from build123d import *

# Parameters (mm, degrees)
BOSS_EXTRUDE2_DEPTH = 15
SKETCH4_R           = 5
BOSS_EXTRUDE3_DEPTH = 55
SKETCH5_R           = 2.5
BOSS_EXTRUDE5_DEPTH = 30
BOSS_EXTRUDE6_START = 20
SKETCH6_R           = 5
BOSS_EXTRUDE6_DEPTH = 20
SKETCH9_R           = 5
BOSS_EXTRUDE7_DEPTH = 20
SKETCH10_R          = 5
SKETCH10_R_2        = 3.5
CUT_EXTRUDE1_DEPTH  = 7


# Read off the part's stored shape, not the designer's step: Boss-Extrude2
with BuildPart() as part:
    # Boss-Extrude2 outline → Boss-Extrude2 (new body)
    with BuildSketch(Plane(origin=(0, 0, 0), x_dir=(1, 0, 0), z_dir=(0, 1, 0))):
        with BuildLine():
            ThreePointArc((-79.301270189, 80.000000278), (-85.640172505, 84.817399775), (-88.584206568, 77.419989152))
            add(Edge.make_bspline(
                [(-88.584206568, 77.419989152), (-86.367928891, 69.782262616), (-83.408582461, 63.514951385)],
                knots=[0.02157692, 0.02157692, 0.02157692, 0.151234515, 0.151234515, 0.151234515], degree=2))
            Line((-83.408582461, 63.514951385), (-110.262794416, 79.019237886))
            Line((-110.262794416, 79.019237886), (-115.262794416, 70.358983849))
            Line((-115.262794416, 70.358983849), (-63.301270189, 40.358983849))
            add(Edge.make_bspline(
                [(-63.301270189, 40.358983849), (-45.646570728, 30.396854404), (-18.218994006, 38.458495307)],
                knots=[0.484299762, 0.484299762, 0.484299762, 0.954512817, 0.954512817, 0.954512817], degree=2))
            ThreePointArc((-18.218994006, 38.458495307), (-3.922368216, 28.792616834), (12.885706155, 32.705589052))
            add(Edge.make_bspline(
                [(29.05383915, 7.474920109), (25.9728438, 20.230319759), (12.885706155, 32.705589052)],
                knots=[0.594463111, 0.594463111, 0.594463111, 0.969398026, 0.969398026, 0.969398026], degree=2))
            ThreePointArc((29.05383915, 7.474920109), (29.76251984, 3.767281878), (30, 0))
            add(Edge.make_bspline(
                [(13.669872981, -33.676914536), (30.204968933, -16.604131181), (30, 0)],
                knots=[0, 0, 0, 0.484954637, 0.484954637, 0.484954637], degree=2))
            ThreePointArc((13.669872981, -33.676914536), (12.667333455, -41.575264764), (20.545696107, -40.426167838))
            add(Edge.make_bspline(
                [(20.545696107, -40.426167838), (26.052022476, -34.6879518), (30, -28.991426998)],
                knots=[0.02157692, 0.02157692, 0.02157692, 0.151234515, 0.151234515, 0.151234515], degree=2))
            Line((30, -28.991426998), (30, -60))
            Line((30, -60), (40, -60))
            Line((40, -60), (40, 0))
            add(Edge.make_bspline(
                [(40, 0), (39.800107444, 20.270482952), (19.104733265, 39.992640706)],
                knots=[0.484299762, 0.484299762, 0.484299762, 0.954512817, 0.954512817, 0.954512817], degree=2))
            ThreePointArc((19.104733265, 39.992640706), (20.327316677, 57.206821065), (8.534546147, 69.80655435))
            add(Edge.make_bspline(
                [(65.631397208, 103.676914536), (19.549675952, 115.237660492), (8.534546147, 69.80655435)],
                knots=[0, 0, 0, 0.969398026, 0.969398026, 0.969398026], degree=2))
            ThreePointArc((65.631397208, 103.676914536), (72.972838916, 106.757864952), (68.038510461, 113.006178686))
            add(Edge.make_bspline(
                [(68.038510461, 113.006178686), (60.315906416, 114.905689184), (53.408582461, 115.476475612)],
                knots=[0.02157692, 0.02157692, 0.02157692, 0.151234515, 0.151234515, 0.151234515], degree=2))
            Line((53.408582461, 115.476475612), (80.262794416, 130.980762114))
            Line((80.262794416, 130.980762114), (75.262794416, 139.641016151))
            Line((75.262794416, 139.641016151), (23.301270189, 109.641016151))
            add(Edge.make_bspline(
                [(23.301270189, 109.641016151), (5.846463284, 99.332662644), (-0.885739259, 71.548863987)],
                knots=[0.484299762, 0.484299762, 0.484299762, 0.954512817, 0.954512817, 0.954512817], degree=2))
            ThreePointArc((-0.885739259, 71.548863987), (-16.404948461, 64.000562101), (-21.420252302, 47.487856599))
            add(Edge.make_bspline(
                [(-79.301270189, 80.000000278), (-66.272309422, 34.311685724), (-21.420252302, 47.487856599)],
                knots=[0, 0, 0, 0.969398026, 0.969398026, 0.969398026], degree=2))
        make_face()
    extrude(amount=BOSS_EXTRUDE2_DEPTH)

    # Sketch4 → Boss-Extrude3 (add)
    with BuildSketch(Plane.XZ):
        with Locations(Location((-108.432667397, -72.189110868, 0), (0, 0, 120))):
            Circle(SKETCH4_R)
        with Locations(Location((35, 55, 0), (0, 0, 90))):
            Circle(SKETCH4_R)
        with Locations(Location((73.432667397, -132.810889132, 0), (0, 0, 60))):
            Circle(SKETCH4_R)
    extrude(amount=BOSS_EXTRUDE3_DEPTH)

    # Sketch5 → Boss-Extrude5 (add)
    with BuildSketch(Plane.XZ.offset(55)):
        with Locations(Location((35, 55, 0), (0, 0, 270))):
            Circle(SKETCH5_R)
        with Locations(Location((73.432667397, -132.810889132, 0), (0, 0, 270))):
            Circle(SKETCH5_R)
        with Locations(Location((-108.432667397, -72.189110868, 0), (0, 0, 270))):
            Circle(SKETCH5_R)
    extrude(amount=BOSS_EXTRUDE5_DEPTH)

    # Sketch6 → Boss-Extrude6 (add)
    with BuildSketch(Plane.XZ.offset(BOSS_EXTRUDE6_START)):
        with Locations(Location((16.169872981, 38.007041555, 0), (0, 0, 270))):
            Circle(SKETCH6_R)
        with Locations(Location((-84.301270189, -80, 0), (0, 0, 270))):
            Circle(SKETCH6_R)
        with Locations(Location((68.131397208, -108.007041555, 0), (0, 0, 270))):
            Circle(SKETCH6_R)
    extrude(amount=-BOSS_EXTRUDE6_DEPTH)

    # Sketch9 → Boss-Extrude7 (add)
    with BuildSketch(Plane.XZ):
        with Locations(Location((-15.107039064, -44.643969537, 0), (0, 0, 90))):
            Circle(SKETCH9_R)
        with Locations(Location((12.191977977, -39.594935626, 0), (0, 0, 90))):
            Circle(SKETCH9_R)
        with Locations(Location((2.915061087, -65.761094837, 0), (0, 0, 90))):
            Circle(SKETCH9_R)
    extrude(amount=BOSS_EXTRUDE7_DEPTH)

    # Sketch10 → Cut-Extrude1 (cut)
    # profile 1 of 6: a face of its own
    with BuildSketch(Plane(origin=(0, -20, 0), x_dir=(-1, 0, 0), z_dir=(0, -1, 0))):
        with Locations(Location((-16.169872981, -38.007041555, 0), (0, 0, 90))):
            Circle(SKETCH10_R)
        with Locations(Location((-16.169872981, -38.007041555, 0), (0, 0, 90))):
            Circle(SKETCH10_R_2, mode=Mode.SUBTRACT)
    # profile 2 of 6: a face of its own
    with BuildSketch(Plane(origin=(0, -20, 0), x_dir=(-1, 0, 0), z_dir=(0, -1, 0))):
        with Locations(Location((-68.131397208, 108.007041555, 0), (0, 0, 90))):
            Circle(SKETCH10_R)
        with Locations(Location((-68.131397208, 108.007041555, 0), (0, 0, 90))):
            Circle(SKETCH10_R_2, mode=Mode.SUBTRACT)
    # profile 3 of 6: a face of its own
    with BuildSketch(Plane(origin=(0, -20, 0), x_dir=(-1, 0, 0), z_dir=(0, -1, 0))):
        with Locations(Location((-12.191977977, 39.594935626, 0), (0, 0, 270))):
            Circle(SKETCH10_R)
        with Locations(Location((-12.191977977, 39.594935626, 0), (0, 0, 90))):
            Circle(SKETCH10_R_2, mode=Mode.SUBTRACT)
    # profile 4 of 6: a face of its own
    with BuildSketch(Plane(origin=(0, -20, 0), x_dir=(-1, 0, 0), z_dir=(0, -1, 0))):
        with Locations(Location((-2.915061087, 65.761094837, 0), (0, 0, 270))):
            Circle(SKETCH10_R)
        with Locations(Location((-2.915061087, 65.761094837, 0), (0, 0, 90))):
            Circle(SKETCH10_R_2, mode=Mode.SUBTRACT)
    # profile 5 of 6: a face of its own
    with BuildSketch(Plane(origin=(0, -20, 0), x_dir=(-1, 0, 0), z_dir=(0, -1, 0))):
        with Locations(Location((15.107039064, 44.643969537, 0), (0, 0, 270))):
            Circle(SKETCH10_R)
        with Locations(Location((15.107039064, 44.643969537, 0), (0, 0, 90))):
            Circle(SKETCH10_R_2, mode=Mode.SUBTRACT)
    # profile 6 of 6: a face of its own
    with BuildSketch(Plane(origin=(0, -20, 0), x_dir=(-1, 0, 0), z_dir=(0, -1, 0))):
        with Locations(Location((84.301270189, 80, 0), (0, 0, 90))):
            Circle(SKETCH10_R)
        with Locations(Location((84.301270189, 80, 0), (0, 0, 90))):
            Circle(SKETCH10_R_2, mode=Mode.SUBTRACT)
    extrude(amount=-CUT_EXTRUDE1_DEPTH, mode=Mode.SUBTRACT)


solid = part.part
Verification items for the finished model (mm, model axes). A direction names the side the tool comes from. Give positions to 0.01 mm unless a question says otherwise; leave off trailing zeros. Write each loop counter-clockwise with the first axis right and the second up, starting at its lowest first coordinate (ties: lowest second). Pieces come first, ordered by that corner, then holes. Notation, with made-up numbers: M 57,83.25 L 115,83.25 A8 cw 115,88.25 Z; hole C -21.5,27 d11. An arc over 180 degrees is marked long. Put each result on its own line as item: value. Start each with the question number.
1. Draft check along X on faces 1 (the face through (73, -85, -133)), 2 (the face through (-110.873, -69.79, -71.647)), 3 (the face through (30, 7, 44)). Enter one of: +X half, -X half, draft (parallel to the pull), parting line (faces both ways), or undercut.
2. Section check C-C (y = -79). Record the cut outline in (x, z), and give its area (3 significant figures).
3. Section check A-A (y = -10.5). Give the number of separate pieces and of enclosed holes in the cut face, and give its area (3 significant figures).
4. Go/stop test with flat-tipped pins: pin 1 Ø5 at (x, z) = (14, -38) entering from -Y; pin 2 Ø7.5 at (y, z) = (8, 42) entering from -X; pin 3 Ø5.5 at (x, z) = (36.5, 57.5) entering from -Y; pin 4 Ø1.3 at (x, z) = (-110, -76) entering from -Y. Record where each tip stops, or that it passes through.
5. Set-up check for faces 4 (the face through (3, -20, -66)), 5 (the face through (39, 0, 59)), 6 (the face through (-12.06, -6.41, -48.61)), 7 (the face through (31, 0, 59)): record each of +Z, -Z, +X, -X, +Y, -Y from which the full face is reachable in a straight line by a thin tool's end or side.
6. Scan lines: line 1 along Z through (x, y) = (26, 1); line 2 along X through (y, z) = (-45, -128.5); line 3 along Y through (x, z) = (-6, -41.5). Record each from-to range of solid material in increasing order. Write a range as [from, to].
7. Section check B-B (y = -44.5). Record the cut outline in (x, z).
Answer list:
1. face 1: draft
1. face 2: parting line
1. face 3: undercut
2. outline: C -108.43,-72.19 d5; C 35,55 d5; C 73.43,-132.81 d5
2. area: 58.9 mm2
3. separate pieces: 9
3. enclosed holes: 0
3. area: 707 mm2
4. pin 1: y = -20
4. pin 2: x = 11.18
4. pin 3: y = -85
4. pin 4: y = -55
5. face 4: +Z, -Z, +X, -Y
5. face 5: +Z, +X, -Y
5. face 6: -Y
5. face 7: +Z, -X, -Y
6. line 1: [-111.2, -99.48], [-32.75, -15.72], [16.76, 34.29]
6. line 2: [70.9, 75.97]
6. line 3: [0, 15]
7. outline: C -108.43,-72.19 d10; C 35,55 d10; C 73.43,-132.81 d10
